from build123d import *

# Parameters (mm, degrees)
SKETCH1_R               = 9
BOSS_EXTRUDE1_DEPTH     = 18
CUT_EXTRUDE1_DEPTH      = 23.045407685
CUT_EXTRUDE1_DEPTH_BACK = 23.045407685
SKETCH4_R               = 5.5
SKETCH2_R               = 2.5
CUT_EXTRUDE2_DEPTH      = 5
CUT_EXTRUDE6_START      = -1
CUT_EXTRUDE6_DEPTH      = 2
SKETCH8_R               = 5
BOSS_EXTRUDE2_DEPTH     = 10


with BuildPart() as part:
    # Sketch1 → Boss-Extrude1 (new body)
    with BuildSketch(Plane(origin=(0, 0, 0), x_dir=(1, 0, 0), z_dir=(0, 1, 0))):
        with Locations(Location((0, 0, 0), (0, 0, 270))):
            Circle(SKETCH1_R)
    extrude(amount=BOSS_EXTRUDE1_DEPTH)

    # Sketch4 → Cut-Extrude1 (cut, two sides: drawn at the far end of the back side and taken through both)
    with BuildSketch(Plane(origin=(0, 0, 0), x_dir=(0, 0, -1), z_dir=(1, 0, 0)).offset(-CUT_EXTRUDE1_DEPTH_BACK)):
        with Locations((0, 10)):
            Circle(SKETCH4_R)
    extrude(amount=CUT_EXTRUDE1_DEPTH + CUT_EXTRUDE1_DEPTH_BACK, mode=Mode.SUBTRACT)

    # Sketch2 → Cut-Extrude2 (cut)
    with BuildSketch(Plane(origin=(0, 18, 0), x_dir=(1, 0, 0), z_dir=(0, 1, 0))):
        with Locations(Location((0, 0, 0), (0, 0, 270))):
            Circle(SKETCH2_R)
    extrude(amount=-CUT_EXTRUDE2_DEPTH, mode=Mode.SUBTRACT)

    # Sketch7 → Cut-Extrude6 (cut)
    with BuildSketch(Plane(origin=(0, 18, 0), x_dir=(1, 0, 0), z_dir=(0, 1, 0)).offset(CUT_EXTRUDE6_START)):
        Polygon((-2.299117574, -1.74567801), (0.362242716, -2.86393323), (2.66136029, -1.118255221), (2.299117574, 1.74567801), (-0.362242716, 2.86393323), (-2.66136029, 1.118255221), align=None)
    extrude(amount=-CUT_EXTRUDE6_DEPTH, mode=Mode.SUBTRACT)

    # Sketch8 → Boss-Extrude2 (add)
    with BuildSketch(Plane.XZ):
        with Locations(Location((0, 0, 0), (0, 0, 270))):
            Circle(SKETCH8_R)
    extrude(amount=BOSS_EXTRUDE2_DEPTH)


solid = part.part
Here's how the part is built. I have some questions about the finished solid (model axes, mm). A direction names the side the tool comes from. Round coordinates to 2 decimals unless told otherwise and drop trailing zeros. Write each loop counter-clockwise with the first axis right and the second up, starting at its lowest first coordinate (ties: lowest second). Pieces come first, ordered by that corner, then holes.
1. I need wall thicknesses on L1, parallel to Z at x = -4, y = 10; L2, parallel to Y at x = 3.75, z = -1; L3, parallel to X at y = 17.45, z = 0. Which ranges of each line are inside material? Lowest first, please.
2. For faces 1 (the cylindrical face through (-4.88, -4.93, 1.08)), 2 (the flat face through (0.987, 16.014, -2.297)), 3 (the cylindrical face through (-2.44, 17.51, -0.54)), which set-ups out of +Z, -Z, +X, -X, +Y, -Y let a thin tool reach every point of the face, with its end or its side?
3. If we mould it in two halves opening along Z, with no side actions, what happens to faces 4 (the flat face through (-2.12, 17, 1.6)), 5 (the flat face through (-2, 18, 2)), 6 (the cylindrical face through (6.083, 8.874, -6.633))? For each: released by +Z, released by -Z, zero draft, split by the parting line, or undercut.
4. Suppose I cut it at A-A (x = 3). List the corners of the cut face in (y, z) for me.
5. Suppose I cut it at C-C (y = -1.25). List the corners of the cut face in (x, z) for me.
6. Suppose I cut it at B-B (z = 0). State how many separate pieces and enclosed holes the cut face has, and give its area (3 significant figures).
7. Suppose I cut it at D-D (x = 0). List the corners of the cut face in (y, z) for me.
8. Will these pins go through, and if not, where does the flat tip stop? pin 1 Ø1 at (x, z) = (0, -1) entering from +Y; pin 2 Ø2 at (x, y) = (-3, -4) entering from +Z; pin 3 Ø8 at (y, z) = (-7, 3) entering from +X.
Answer sheet:
1. L1: z = -8.06 to -5.5, 5.5 to 8.06
1. L2: y = -10 to 4.59, 15.41 to 18
1. L3: x = -9 to -2.5, 2.5 to 9
2. face 1: -Y
2. face 2: none
2. face 3: +Y
3. face 4: undercut
3. face 5: zero draft
3. face 6: split by the parting line
4. outline: (-10, -4) - (0, -4) - (0, -8.49) - (18, -8.49) - (18, 8.49) - (0, 8.49) - (0, 4) - (-10, 4) - close; hole circle Ø11 at (10, 0)
5. outline: circle Ø10 at (0, 0)
6. separate pieces: 3
6. enclosed holes: 0
6. area: 213 mm2
7. outline: (-10, -5) - (0, -5) - (0, -9) - (18, -9) - (18, -2.5) - (17, -2.5) - (17, -2.71) - (15, -2.71) - (15, -2.5) - (14.9, -2.5) arc R5.5 cw (long way) to (14.9, 2.5) - (15, 2.5) - (15, 2.71) - (17, 2.71) - (17, 2.5) - (18, 2.5) - (18, 9) - (0, 9) - (0, 5) - (-10, 5) - close
8. pin 1: stops at y = 4.71
8. pin 2: stops at z = 4.58
8. pin 3: stops at x = 5
